Geometry check sheet. Reference: the model listing, model coordinates, mm. A direction names the side the tool comes from. Coordinates: 2 decimals unless noted, no trailing zeros. Write each loop counter-clockwise with the first axis right and the second up, starting at its lowest first coordinate (ties: lowest second). Pieces come first, ordered by that corner, then holes. Notation, with made-up numbers: M -26.75,45 L 7.25,45 A29 ccw 7.25,66 Z; hole C -1,46.5 d7. An arc over 180 degrees is marked long. Write each question's results on one line, items separated by ' | '.
```python
from build123d import *

# Parameters (mm, degrees)
SKETCH_1_R          = 2
SKETCH_1_W          = 35
SKETCH_1_H          = 3
SKETCH_1_H_2        = 40
SKETCH_1_R_2        = 45
EXTRUDE_3_DEPTH     = 4
FILLET_1_R          = 8
SKETCH_4_R          = 2
CUT_EXTRUDE_3_DEPTH = 4
SKETCH_6_R          = 2
CUT_EXTRUDE_5_DEPTH = 10
SKETCH_7_W          = 80
SKETCH_7_H          = 100
CUT_EXTRUDE_6_DEPTH = 10
FILLET_2_R          = 10
SKETCH_8_W          = 3
SKETCH_8_H          = 7
EXTRUDE_5_DEPTH     = 4
SKETCH_8_4_W        = 5
SKETCH_8_4_H        = 7
CUT_EXTRUDE_7_DEPTH = 4
SKETCH_9_W          = 2
SKETCH_9_H          = 3
SKETCH_9_H_2        = 40
CUT_EXTRUDE_8_DEPTH = 4
FILLET_3_R          = 1


with BuildPart() as part:
    # Sketch 1 → Extrude 3 (new body)
    with BuildSketch(Plane.XY):
        Polygon((123.0688133, -57.848092329), (123.0688133, 62.151907671), (73.0688133, 62.151907671), (73.0688133, 142.151907671), (-86.9311867, 142.151907671), (-86.9311867, 62.151907671), (-136.9311867, 62.151907671), (-136.9311867, -57.848092329), (-86.9311867, -57.848092329), (-86.9311867, -137.848092329), (73.0688133, -137.848092329), (73.0688133, -57.848092329), align=None)
        with Locations((-71.9311867, -82.848092329)):
            Circle(SKETCH_1_R, mode=Mode.SUBTRACT)
        with Locations((-71.9311867, -112.848092329)):
            Circle(SKETCH_1_R, mode=Mode.SUBTRACT)
        with Locations((-64.4311867, -130.848092329)):
            Circle(SKETCH_1_R, mode=Mode.SUBTRACT)
        with Locations((-31.9311867, -129.848092329)):
            Circle(SKETCH_1_R, mode=Mode.SUBTRACT)
        with Locations((18.0688133, -129.848092329)):
            Circle(SKETCH_1_R, mode=Mode.SUBTRACT)
        with Locations((50.5688133, -130.848092329)):
            Circle(SKETCH_1_R, mode=Mode.SUBTRACT)
        with Locations((58.0688133, -112.848092329)):
            Circle(SKETCH_1_R, mode=Mode.SUBTRACT)
        with Locations((58.0688133, -82.848092329)):
            Circle(SKETCH_1_R, mode=Mode.SUBTRACT)
        with Locations((50.5688133, -64.848092329)):
            Circle(SKETCH_1_R, mode=Mode.SUBTRACT)
        with Locations((-64.4311867, -64.848092329)):
            Circle(SKETCH_1_R, mode=Mode.SUBTRACT)
        with Locations((34.0688133, -112.848092329)):
            Circle(SKETCH_1_R, mode=Mode.SUBTRACT)
        with Locations((34.0688133, -82.848092329)):
            Circle(SKETCH_1_R, mode=Mode.SUBTRACT)
        with Locations((-31.9311867, -79.848092329)):
            Circle(SKETCH_1_R, mode=Mode.SUBTRACT)
        with Locations((18.0688133, -79.848092329)):
            Circle(SKETCH_1_R, mode=Mode.SUBTRACT)
        with Locations((-47.9311867, -82.848092329)):
            Circle(SKETCH_1_R, mode=Mode.SUBTRACT)
        with Locations((-47.9311867, -112.848092329)):
            Circle(SKETCH_1_R, mode=Mode.SUBTRACT)
        with Locations((-107.4311867, 16.401907671)):
            Rectangle(SKETCH_1_W, SKETCH_1_H, mode=Mode.SUBTRACT)
        with Locations((-107.4311867, -7.848092329)):
            Rectangle(SKETCH_1_W, SKETCH_1_H_2, mode=Mode.SUBTRACT)
        with Locations((-107.4311867, -32.098092329)):
            Rectangle(SKETCH_1_W, SKETCH_1_H, mode=Mode.SUBTRACT)
        with Locations((103.0688133, 37.151907671)):
            Circle(SKETCH_1_R, mode=Mode.SUBTRACT)
        with Locations((103.0688133, -32.848092329)):
            Circle(SKETCH_1_R, mode=Mode.SUBTRACT)
        with Locations((68.0688133, 2.151907671)):
            Circle(SKETCH_1_R_2, mode=Mode.SUBTRACT)
        with Locations((33.0688133, -32.848092329)):
            Circle(SKETCH_1_R, mode=Mode.SUBTRACT)
        with Locations((33.0688133, 37.151907671)):
            Circle(SKETCH_1_R, mode=Mode.SUBTRACT)
        with Locations((50.5688133, 135.151907671)):
            Circle(SKETCH_1_R, mode=Mode.SUBTRACT)
        with Locations((58.0688133, 117.151907671)):
            Circle(SKETCH_1_R, mode=Mode.SUBTRACT)
        with Locations((58.0688133, 87.151907671)):
            Circle(SKETCH_1_R, mode=Mode.SUBTRACT)
        with Locations((34.0688133, 87.151907671)):
            Circle(SKETCH_1_R, mode=Mode.SUBTRACT)
        with Locations((34.0688133, 117.151907671)):
            Circle(SKETCH_1_R, mode=Mode.SUBTRACT)
        with Locations((50.5688133, 69.151907671)):
            Circle(SKETCH_1_R, mode=Mode.SUBTRACT)
        with Locations((-64.4311867, 69.151907671)):
            Circle(SKETCH_1_R, mode=Mode.SUBTRACT)
        with Locations((-71.9311867, 87.151907671)):
            Circle(SKETCH_1_R, mode=Mode.SUBTRACT)
        with Locations((-71.9311867, 117.151907671)):
            Circle(SKETCH_1_R, mode=Mode.SUBTRACT)
        with Locations((-47.9311867, 117.151907671)):
            Circle(SKETCH_1_R, mode=Mode.SUBTRACT)
        with Locations((-47.9311867, 87.151907671)):
            Circle(SKETCH_1_R, mode=Mode.SUBTRACT)
        with Locations((-64.4311867, 135.151907671)):
            Circle(SKETCH_1_R, mode=Mode.SUBTRACT)
    extrude(amount=EXTRUDE_3_DEPTH)

    # Fillet 1
    fillet_1_edges = [part.edges().sort_by_distance(p)[0] for p in [
        (73.0688133, -137.848092329, 2),
        (-86.9311867, -137.848092329, 2),
        (-136.9311867, -57.848092329, 2),
        (-136.9311867, 62.151907671, 2),
        (-86.9311867, 142.151907671, 2),
        (73.0688133, 142.151907671, 2),
        (123.0688133, 62.151907671, 2),
        (123.0688133, -57.848092329, 2),
    ]]
    fillet(fillet_1_edges, radius=FILLET_1_R)

    # Sketch 4 → Cut-Extrude 3 (cut)
    with BuildSketch(Plane.XY.offset(4)):
        with Locations((-129.9311867, 55.151907671)):
            Circle(SKETCH_4_R)
        with Locations((-129.9311867, -50.848092329)):
            Circle(SKETCH_4_R)
        with Locations((116.0688133, 55.151907671)):
            Circle(SKETCH_4_R)
        with Locations((116.0688133, -50.848092329)):
            Circle(SKETCH_4_R)
        with Locations((-24.9311867, 135.151907671)):
            Circle(SKETCH_4_R)
        with Locations((11.0688133, 135.151907671)):
            Circle(SKETCH_4_R)
        with Locations((-24.9311867, -130.848092329)):
            Circle(SKETCH_4_R)
        with Locations((11.0688133, -130.848092329)):
            Circle(SKETCH_4_R)
    extrude(amount=-CUT_EXTRUDE_3_DEPTH, mode=Mode.SUBTRACT)

    # Sketch 6 → Cut-Extrude 5 (cut)
    with BuildSketch(Plane.XY.offset(4)):
        with Locations((-31.9311867, 134.151907671)):
            Circle(SKETCH_6_R)
        with Locations((18.0688133, 134.151907671)):
            Circle(SKETCH_6_R)
        with Locations((-31.9311867, 84.151907671)):
            Circle(SKETCH_6_R)
        with Locations((18.0688133, 84.151907671)):
            Circle(SKETCH_6_R)
    extrude(amount=-CUT_EXTRUDE_5_DEPTH, mode=Mode.SUBTRACT)

    # Sketch 7 → Cut-Extrude 6 (cut)
    with BuildSketch(Plane.XY.offset(4)):
        with Locations((-30.9311867, 2.151907671)):
            Rectangle(SKETCH_7_W, SKETCH_7_H)
    extrude(amount=-CUT_EXTRUDE_6_DEPTH, mode=Mode.SUBTRACT)

    # Fillet 2
    fillet_2_edges = [part.edges().sort_by_distance(p)[0] for p in [
        (-70.9311867, -47.848092329, 2),
        (-70.9311867, 52.151907671, 2),
        (9.0688133, 52.151907671, 2),
        (9.0688133, -47.848092329, 2),
    ]]
    fillet(fillet_2_edges, radius=FILLET_2_R)

    # Sketch 8 → Extrude 5 (add)
    with BuildSketch(Plane(origin=(0, 0, 0), x_dir=(-1, 0, 0), z_dir=(0, 0, -1))):
        Polygon((86.9311867, 19.151907671), (86.9311867, 12.151907671), (89.9311867, 12.151907671), (94.4311867, 12.151907671), (94.4311867, 19.151907671), align=None)
        Polygon((86.9311867, -33.598092329), (102.4311867, -33.598092329), (102.4311867, -27.848092329), (89.9311867, -27.848092329), (89.9311867, 12.151907671), (86.9311867, 12.151907671), align=None)
        with Locations((100.9311867, 15.651907671)):
            Rectangle(SKETCH_8_W, SKETCH_8_H)
    extrude(amount=-EXTRUDE_5_DEPTH)

    # Sketch 8_4 → Cut-Extrude 7 (cut)
    with BuildSketch(Plane(origin=(0, 0, 0), x_dir=(-1, 0, 0), z_dir=(0, 0, -1))):
        with Locations((96.9311867, 15.651907671)):
            Rectangle(SKETCH_8_4_W, SKETCH_8_4_H)
    extrude(amount=-CUT_EXTRUDE_7_DEPTH, mode=Mode.SUBTRACT)

    # Sketch 9 → Cut-Extrude 8 (cut)
    with BuildSketch(Plane(origin=(0, 0, 0), x_dir=(-1, 0, 0), z_dir=(0, 0, -1))):
        with Locations((125.9311867, 16.401907671)):
            Rectangle(SKETCH_9_W, SKETCH_9_H)
        with Locations((125.9311867, -32.098092329)):
            Rectangle(SKETCH_9_W, SKETCH_9_H)
        with Locations((125.9311867, -7.848092329)):
            Rectangle(SKETCH_9_W, SKETCH_9_H_2)
    extrude(amount=-CUT_EXTRUDE_8_DEPTH, mode=Mode.SUBTRACT)

    # Fillet 3
    fillet_3_edges = [part.edges().sort_by_distance(p)[0] for p in [
        (-99.4311867, 12.151907671, 2),
        (-94.4311867, 12.151907671, 2),
    ]]
    fillet(fillet_3_edges, radius=FILLET_3_R)


solid = part.part
```
Q1. Depth check by flat-ended pin: P1, Ø1.2, axis at y = 96.5, z = 2, coming from the +X side; P2, Ø1.2, axis at x = -119.5, z = 2.5, coming from the -Y side; P3, Ø2, axis at y = -78.5, z = 2, coming from the -X side. Enter the tip coordinate at first touch or a pass-through.
Geometry check:
P1: stops at x = 73.07 | P2: stops at y = -57.85 | P3: stops at x = -86.93
Q2. Sectioned sample at A-A on x = -117. Record the cut outline in (y, z), and give its area (3 significant figures).
Geometry check:
outline: M -57.85,0 L -33.6,0 L -33.6,4 L -57.85,4 Z; M -30.6,0 L -27.85,0 L -27.85,4 L -30.6,4 Z; M 12.15,0 L 14.9,0 L 14.9,4 L 12.15,4 Z; M 17.9,0 L 62.15,0 L 62.15,4 L 17.9,4 Z | area: 296 mm2
Q3. Sectioned sample at D-D on z = 2. Give the number of separate pieces and of enclosed holes in the cut face, and give its area (3 significant figures).
Geometry check:
separate pieces: 1 | enclosed holes: 49 | area: 40,200 mm2
Q4. Sectioned sample at C-C on y = -7.5. Record the cut outline in (x, z), and give its area (3 significant figures).
Geometry check:
outline: M -136.93,0 L -126.93,0 L -126.93,4 L -136.93,4 Z; M -89.93,0 L -70.93,0 L -70.93,4 L -89.93,4 Z; M 9.07,0 L 24.12,0 L 24.12,4 L 9.07,4 Z; M 112.02,0 L 123.07,0 L 123.07,4 L 112.02,4 Z | area: 220 mm2
Q5. Access from +Z, -Z, +X, -X, +Y, -Y to the whole of each face (thin tool, end or side, straight path). Record for faces 4 (the cylindrical face through (6.22, 49.14, 1.97)), 5 (the cylindrical face through (-134.525, 59.871, 2.028)).
Geometry check:
face 4: +Z, -Z | face 5: +Z, -Z, -X, +Y
Q6. Scan lines: probe 1 along X at (y, z) = (4, 1.55); probe 2 along Y at (x, z) = (-126, 1.65); probe 3 along Y at (x, z) = (-60, 0.4). Record each from-to range of solid material in increasing order.
Geometry check:
probe 1: x = -136.93 to -126.93, -89.93 to -70.93, 9.07 to 23.11, 113.03 to 123.07 | probe 2: y = -57.85 to -33.6, -30.6 to -27.85, 12.15 to 14.9, 17.9 to 62.15 | probe 3: y = -137.85 to -47.85, 52.15 to 142.15
Q7. Mould release check, pull along Y, two halves, no side actions. Record for faces 1 (the cylindrical face through (6.06, -45, 1.97)), 2 (the cylindrical face through (70.788, 139.746, 2.028)), 3 (the flat face through (20, 4, 0)): pulls with the +Y half, pulls with the -Y half, needs draft (parallel to the pull), parting line crosses it, or undercut.
Geometry check:
face 1: undercut | face 2: pulls with the +Y half | face 3: needs draft
Q8. Sectioned sample at B-B on x = 5.5. Record the cut outline in (y, z), and give its area (3 significant figures).
Geometry check:
outline: M -137.85,0 L -45.51,0 L -45.51,4 L -137.85,4 Z; M 49.81,0 L 142.15,0 L 142.15,4 L 49.81,4 Z | area: 739 mm2
